from build123d import *

# Parameters (mm, degrees)
SKETCH_1_R      = 2.2
EXTRUDE_1_DEPTH = 2


with BuildPart() as part:
    # 草图1 → 凸台-拉伸1 (new body)
    with BuildSketch(Plane(origin=(0, 0, 0), x_dir=(1, 0, 0), z_dir=(0, 1, 0))):
        Polygon((159.754738648, 48.995603023), (150.004738648, 48.995603023), (150.004738648, 46.495603023), (151.504738648, 46.495603023), (151.504738648, 43.895603023), (150.004738648, 43.895603023), (150.004738648, 40.895603023), (147.004738648, 40.895603023), (147.004738648, 43.895603023), (145.504738648, 43.895603023), (145.504738648, 46.495603023), (147.004738648, 46.495603023), (147.004738648, 48.995603023), (138.604738648, 48.995603023), (133.504738648, 48.995603023), (118.504738648, 48.995603023), (118.504738648, 33.995603023), (118.504738648, 21.495603023), (118.504738648, 20.495603023), (121.004738648, 20.495603023), (121.004738648, 21.995603023), (123.604738648, 21.995603023), (123.604738648, 20.495603023), (126.604738648, 20.495603023), (126.604738648, 17.495603023), (123.604738648, 17.495603023), (123.604738648, 15.995603023), (121.004738648, 15.995603023), (121.004738648, 17.495603023), (118.504738648, 17.495603023), (118.504738648, 7.745603023), (116.504738648, 7.745603023), (116.504738648, -0.254396977), (118.504738648, -0.254396977), (118.504738648, -27.754396977), (116.504738648, -27.754396977), (116.504738648, -35.754396977), (118.504738648, -35.754396977), (118.504738648, -45.504396977), (121.004738648, -45.504396977), (121.004738648, -44.004396977), (123.604738648, -44.004396977), (123.604738648, -45.504396977), (126.604738648, -45.504396977), (126.604738648, -48.504396977), (123.604738648, -48.504396977), (123.604738648, -50.004396977), (121.004738648, -50.004396977), (121.004738648, -48.504396977), (118.504738648, -48.504396977), (118.504738648, -56.904396977), (118.504738648, -62.004396977), (118.504738648, -77.004396977), (133.504738648, -77.004396977), (146.004738648, -77.004396977), (147.004738648, -77.004396977), (147.004738648, -74.504396977), (145.504738648, -74.504396977), (145.504738648, -71.904396977), (147.004738648, -71.904396977), (147.004738648, -68.904396977), (150.004738648, -68.904396977), (150.004738648, -71.904396977), (151.504738648, -71.904396977), (151.504738648, -74.504396977), (150.004738648, -74.504396977), (150.004738648, -77.004396977), (159.754738648, -77.004396977), (159.754738648, -79.004396977), (167.754738648, -79.004396977), (167.754738648, -77.004396977), (195.254738648, -77.004396977), (195.254738648, -79.004396977), (203.254738648, -79.004396977), (203.254738648, -77.004396977), (213.004738648, -77.004396977), (213.004738648, -74.504396977), (211.504738648, -74.504396977), (211.504738648, -71.904396977), (213.004738648, -71.904396977), (213.004738648, -68.904396977), (216.004738648, -68.904396977), (216.004738648, -71.904396977), (217.504738648, -71.904396977), (217.504738648, -74.504396977), (216.004738648, -74.504396977), (216.004738648, -77.004396977), (224.404738648, -77.004396977), (229.504738648, -77.004396977), (244.504738648, -77.004396977), (244.504738648, -62.004396977), (244.504738648, -49.504396977), (244.504738648, -48.504396977), (242.004738648, -48.504396977), (242.004738648, -50.004396977), (239.404738648, -50.004396977), (239.404738648, -48.504396977), (236.404738648, -48.504396977), (236.404738648, -45.504396977), (239.404738648, -45.504396977), (239.404738648, -44.004396977), (242.004738648, -44.004396977), (242.004738648, -45.504396977), (244.504738648, -45.504396977), (244.504738648, -35.754396977), (246.504738648, -35.754396977), (246.504738648, -27.754396977), (244.504738648, -27.754396977), (244.504738648, -0.254396977), (246.504738648, -0.254396977), (246.504738648, 7.745603023), (244.504738648, 7.745603023), (244.504738648, 17.495603023), (242.004738648, 17.495603023), (242.004738648, 15.995603023), (239.404738648, 15.995603023), (239.404738648, 17.495603023), (236.404738648, 17.495603023), (236.404738648, 20.495603023), (239.404738648, 20.495603023), (239.404738648, 21.995603023), (242.004738648, 21.995603023), (242.004738648, 20.495603023), (244.504738648, 20.495603023), (244.504738648, 28.895603023), (244.504738648, 33.995603023), (244.504738648, 48.995603023), (229.504738648, 48.995603023), (217.004738648, 48.995603023), (216.004738648, 48.995603023), (216.004738648, 46.495603023), (217.504738648, 46.495603023), (217.504738648, 43.895603023), (216.004738648, 43.895603023), (216.004738648, 40.895603023), (213.004738648, 40.895603023), (213.004738648, 43.895603023), (211.504738648, 43.895603023), (211.504738648, 46.495603023), (213.004738648, 46.495603023), (213.004738648, 48.995603023), (203.254738648, 48.995603023), (203.254738648, 50.995603023), (195.254738648, 50.995603023), (195.254738648, 48.995603023), (167.754738648, 48.995603023), (167.754738648, 50.995603023), (159.754738648, 50.995603023), align=None)
        with Locations(Location((181.504738648, -56.504396977, 0), (0, 0, 270))):
            Circle(SKETCH_1_R, mode=Mode.SUBTRACT)
        with Locations(Location((151.452700448, -44.056435178, 0), (0, 0, 270))):
            Circle(SKETCH_1_R, mode=Mode.SUBTRACT)
        with Locations(Location((139.004738648, -14.004396977, 0), (0, 0, 270))):
            Circle(SKETCH_1_R, mode=Mode.SUBTRACT)
        with Locations(Location((224.004738648, -14.004396977, 0), (0, 0, 90))):
            Circle(SKETCH_1_R, mode=Mode.SUBTRACT)
        with Locations(Location((211.556776849, 16.047641223, 0), (0, 0, 270))):
            Circle(SKETCH_1_R, mode=Mode.SUBTRACT)
        with Locations(Location((181.504738648, 28.49819903, 0), (0, 0, 270))):
            Circle(SKETCH_1_R, mode=Mode.SUBTRACT)
        with BuildLine():
            ThreePointArc((156.373636186, -43.170776407), (154.281127573, -41.228008053), (152.338359218, -39.135499439))
            ThreePointArc((152.338359218, -39.135499439), (136.585624733, -32.610503171), (143.110621001, -16.857768685))
            ThreePointArc((143.110621001, -16.857768685), (143.004738648, -14.004396977), (143.110621001, -11.15102527))
            ThreePointArc((143.110621001, -11.15102527), (143.110621001, 24.38972067), (178.65136694, 24.38972067))
            ThreePointArc((178.65136694, 24.38972067), (181.504738648, 24.495603023), (184.358110356, 24.38972067))
            ThreePointArc((184.358110356, 24.38972067), (200.110844842, 30.914716938), (206.63584111, 15.161982452))
            ThreePointArc((206.63584111, 15.161982452), (208.728349724, 13.219214098), (210.671118078, 11.126705484))
            ThreePointArc((210.671118078, 11.126705484), (226.423852564, 4.601709216), (219.898856295, -11.15102527))
            ThreePointArc((219.898856295, -11.15102527), (220.004738648, -14.004396977), (219.898856295, -16.857768685))
            ThreePointArc((219.898856295, -16.857768685), (219.898856295, -52.398514625), (184.358110356, -52.398514625))
            ThreePointArc((184.358110356, -52.398514625), (181.504738648, -52.504396977), (178.65136694, -52.398514625))
            ThreePointArc((178.65136694, -52.398514625), (162.898632455, -58.923510893), (156.373636186, -43.170776407))
        make_face(mode=Mode.SUBTRACT)
    extrude(amount=EXTRUDE_1_DEPTH)


solid = part.part
Here's how the part is built. I have some questions about the finished solid (model axes, mm). A direction names the side the tool comes from. Coordinates: 2 decimals unless noted, no trailing zeros. Write each loop counter-clockwise with the first axis right and the second up, starting at its lowest first coordinate (ties: lowest second). Pieces come first, ordered by that corner, then holes.
1) If we section it at C-C (x = 165): List the corners of the cut face in (y, z) for me.
Filled in:
outline: (0, -51) - (2, -51) - (2, -31.41) - (0, -31.41) - close; (0, 59.58) - (2, 59.58) - (2, 79) - (0, 79) - close
2) If we section it at B-B (x = 187): List the corners of the cut face in (y, z) for me, plus the area to 4 significant figures.
Filled in:
outline: (0, -49) - (2, -49) - (2, -28.33) - (0, -28.33) - close; (0, 54.7) - (2, 54.7) - (2, 77) - (0, 77) - close
area: 85.95 mm2
3) If I drill on line 1 (X direction, y = 1.05, z = -44); line 2 (Z direction, x = 126.5, y = 1.2); line 3 (X direction, y = 0.5, z = 55.5), over which ranges is the centre line in solid material (lowest first)?
Filled in:
line 1: x = 118.5 to 145.5, 151.5 to 211.5, 217.5 to 244.5
line 2: z = -49 to -20.5, -17.5 to 45.5, 48.5 to 77
line 3: x = 118.5 to 158.25, 176.78 to 179.55, 183.46 to 188.13, 216.13 to 244.5
4) If we section it at A-A (z = 56): List the corners of the cut face in (x, y) for me.
Filled in:
outline: (118.5, 0) - (158.69, 0) - (158.69, 2) - (118.5, 2) - close; (176.34, 0) - (179.36, 0) - (179.36, 2) - (176.34, 2) - close; (183.65, 0) - (188.91, 0) - (188.91, 2) - (183.65, 2) - close; (215.35, 0) - (244.5, 0) - (244.5, 2) - (215.35, 2) - close
5) I'm going to push flat-ended pins straight in: pin 1 (0.6 mm diameter, centred on x = 243.5, y = 1.5, fed in from -Z); pin 2 (4 mm diameter, centred on x = 151.45, z = 44.06, fed in from -Y); pin 3 (0.6 mm diameter, centred on x = 119, y = 0.5, fed in from +Z); pin 4 (0.6 mm diameter, centred on x = 117.5, y = 0.5, fed in from -Z). Where does each tip first touch, or does it pass through?
Filled in:
pin 1: stops at z = -49
pin 2: passes through
pin 3: stops at z = 77
pin 4: stops at z = -7.75
6) Which directions (+Z, -Z, +X, -X, +Y, -Y) give clear straight access to the entire face, cutting with the end or side of a thin tool? Please do faces 4 (the face through (208.7, 0.99, -13.25)), 5 (the face through (137, 0, -16)).
Filled in:
face 4: +Y, -Y
face 5: +Z, -Z, +X, -X, -Y
7) If we section it at D-D (y = 1): Count the separate pieces of the cut face and the enclosed holes in it, plus the area to 3 significant figures.
Filled in:
separate pieces: 1
enclosed holes: 7
area: 8,870 mm2
8) Thinking about a two-plate mould opening in Z: for faces 1 (the face through (149.5, 0.99, 45.07)), 2 (the face through (137, 2, -16)), 3 (the face through (179.553, 0.986, -27.483)), which applies, +Z half, -Z half, draft (parallel to the pull), parting line (faces both ways), or undercut?
Filled in:
face 1: undercut
face 2: draft
face 3: undercut
